```python
from build123d import *

# Parameters (mm, degrees)
SKETCH1_R               = 5
BOSS_EXTRUDE1_DEPTH     = 16
SKETCH2_R               = 3.453172081
CUT_EXTRUDE1_DEPTH      = 6
CUT_EXTRUDE1_DEPTH_BACK = 6
CHAMFER1_SIZE           = 1


with BuildPart() as part:
    # Sketch1 → Boss-Extrude1 (new body)
    with BuildSketch(Plane(origin=(0, 0, 0), x_dir=(0, 0, -1), z_dir=(1, 0, 0))):
        Circle(SKETCH1_R)
    extrude(amount=BOSS_EXTRUDE1_DEPTH)

    # Sketch2 → Cut-Extrude1 (cut, two sides)
    with BuildSketch(Plane(origin=(0, 0, 0), x_dir=(1, 0, 0), z_dir=(0, 1, 0))) as cut_extrude1_sk:
        with Locations((8, 0)):
            Circle(SKETCH2_R)
    extrude(amount=CUT_EXTRUDE1_DEPTH, mode=Mode.SUBTRACT)
    extrude(cut_extrude1_sk.sketch, amount=-CUT_EXTRUDE1_DEPTH_BACK, mode=Mode.SUBTRACT)

    # Chamfer1
    chamfer1_edges = [part.edges().sort_by_distance(p)[0] for p in [
        (0, 0, 5),
        (16, 0, 5),
    ]]
    chamfer(chamfer1_edges, length=CHAMFER1_SIZE)


solid = part.part
```
Input: part model. Units: mm. Frame: model coordinates. Round coordinates to 2 decimals unless told otherwise and drop trailing zeros. Loops run counter-clockwise (first coordinate to the right, second up) from the corner with the lowest first, then second, coordinate; pieces in that order, holes last. Notation, with made-up numbers: (30, -13) -> (65, -13) arc R22 cw to (65, -3) -> close; hole circle Ø1 at (81.25, 34.25). An arc over 180 degrees is marked (long way). One line per item, written item: value.
(1) Section C-C (x = 4). Return the cut outline in (y, z).
Geometry check:
outline: circle Ø10 at (0, 0)
(2) Section A-A (z = 0). Return the cut outline in (x, y), plus the area to 3 significant figures.
Geometry check:
outline: (0, -4) -> (1, -5) -> (4.55, -5) -> (4.55, 5) -> (1, 5) -> (0, 4) -> close; (11.45, -5) -> (15, -5) -> (16, -4) -> (16, 4) -> (15, 5) -> (11.45, 5) -> close
area: 88.9 mm2
(3) Section B-B (x = 8). Return the cut outline in (y, z), plus the area to 3 significant figures.
Geometry check:
outline: (-3.62, -3.45) arc R5 ccw to (3.62, -3.45) -> close; (-3.62, 3.45) -> (3.62, 3.45) arc R5 ccw to start
area: 15.4 mm2
(4) Pin query (flat end, axial travel): pin 1 (5 mm diameter, centred on x = 7.5, y = 0.5, fed in from -Z); pin 2 (1.5 mm diameter, centred on x = 10.5, y = -2, fed in from -Z); pin 3 (3 mm diameter, centred on x = 10, z = 3, fed in from -Y); pin 4 (4 mm diameter, centred on x = 7.5, y = 3, fed in from +Z). Return the tip coordinate at first contact, or that it passes through.
Geometry check:
pin 1: z = -5
pin 2: z = -4.84
pin 3: y = -4.66
pin 4: z = 4.9
(5) Material intervals for line 1 (X direction, y = -3.3, z = 0); line 2 (X direction, y = -2.25, z = -1.5); line 3 (Y direction, x = 13.5, z = -3), sorted ascending. Write a range as [from, to].
Geometry check:
line 1: [0, 4.55], [11.45, 16]
line 2: [0, 4.89], [11.11, 16]
line 3: [-4, 4]
